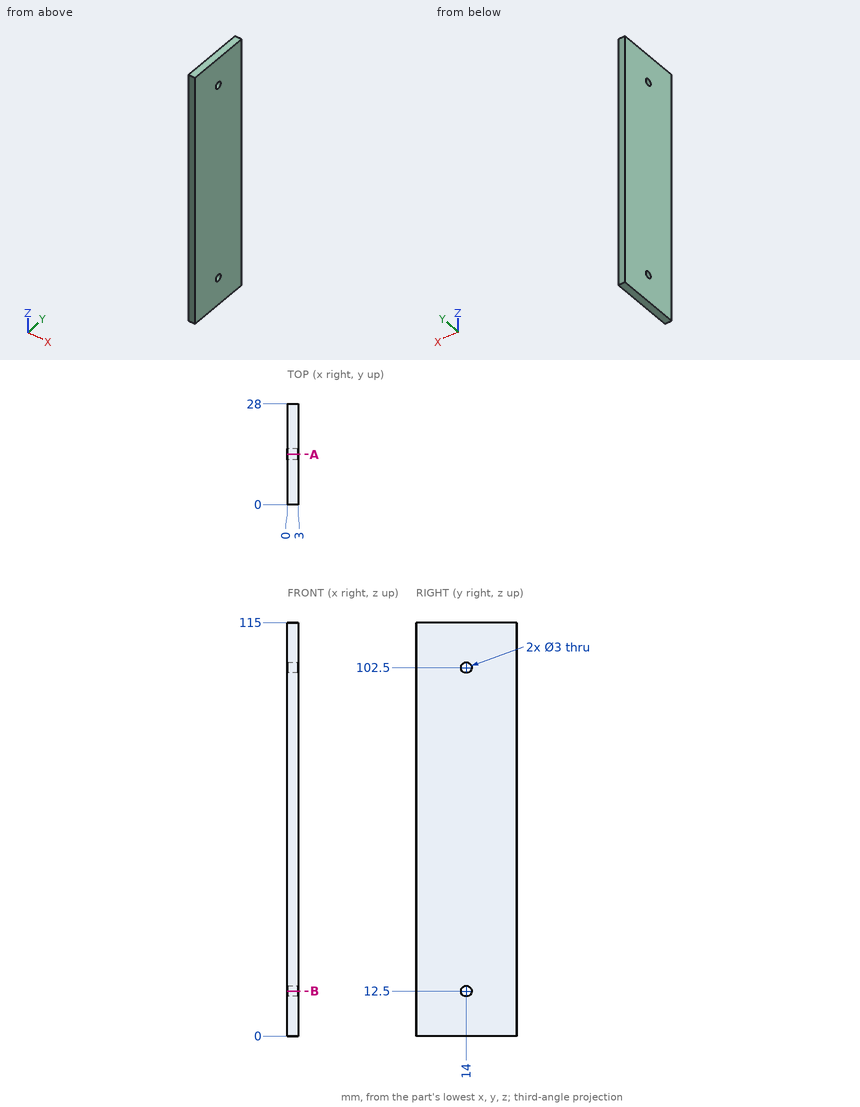
Verification items for this drawing (mm, ordinates from the low corner). Coordinates: 2 decimals unless noted, no trailing zeros. Order: outer loops, then holes, each group sorted by start corner. A loop starts at its lowest first (then second) coordinate and runs counter-clockwise, first axis right, second up. Notation, with made-up numbers: M 1,82 L 54,82 A18 cw 54,93 Z; hole C -6.5,-33.75 d3. An arc over 180 degrees is marked long. Use CSV: the item, a comma, the result in double quotes.
Item 1: Thickness scan on line 1 along Z through (x, y) = (1.85, 14.25); line 2 along Y through (x, z) = (1.65, 102.5); line 3 along Y through (x, z) = (0.55, 103). Record the ranges inside material, lowest first.
Returned:
line 1,"z = 0 to 11.02, 13.98 to 101.02, 103.98 to 115"
line 2,"y = 0 to 12.5, 15.5 to 28"
line 3,"y = 0 to 12.59, 15.41 to 28"
Item 2: Cross-section at A-A on y = 14. Record the cut outline in (x, z), then the cut area to 3 significant figures.
Returned:
outline,"M 0,0 L 3,0 L 3,11 L 0,11 Z; M 0,14 L 3,14 L 3,101 L 0,101 Z; M 0,104 L 3,104 L 3,115 L 0,115 Z"
area,"327 mm2"
Item 3: Cross-section at B-B on z = 12.5. Record the cut outline in (x, y), then the cut area to 3 significant figures.
Returned:
outline,"M 0,0 L 3,0 L 3,12.5 L 0,12.5 Z; M 0,15.5 L 3,15.5 L 3,28 L 0,28 Z"
area,"75.0 mm2"
